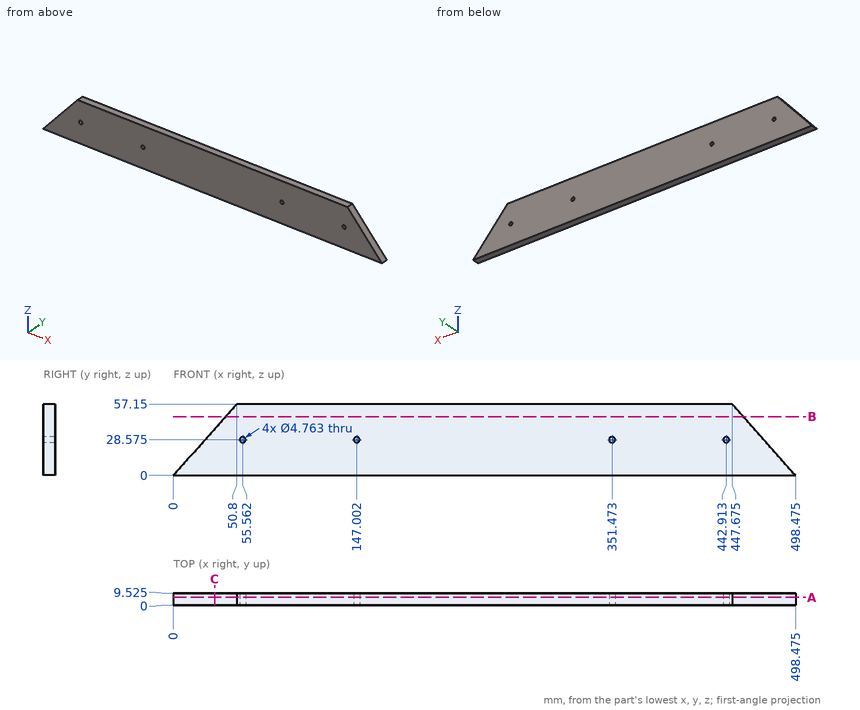
Input: dimensioned drawing with shaded views. Units: mm. Origin: part minimum x, y, z. Give positions to 0.01 mm unless a question says otherwise; leave off trailing zeros. Write each loop counter-clockwise with the first axis right and the second up, starting at its lowest first coordinate (ties: lowest second). Pieces come first, ordered by that corner, then holes. Notation, with made-up numbers: M -40,65 L -13,65 A14 ccw -13,86 Z; hole C -20.75,-21.75 d8. An arc over 180 degrees is marked long. Write item = value, one per line. Start each with the question number.
1) Cut plane A-A on y = 6.25. Count the separate pieces of the cut face and the enclosed holes in it, then the cut area to 3 significant figures.
2) Cut plane C-C on x = 33. Return the cut outline in (y, z) (1 decimal), then the cut area to 3 significant figures.
3) Material intervals for line 1 along X through (y, z) = (2.25, 37.5) (1 decimal); line 2 along X through (y, z) = (5, 22.5) (1 decimal); line 3 along Z through (x, y) = (43.5, 3) (1 decimal), sorted ascending. Write a range as [from, to].
4) First-contact query: pin 1 Ø1 at (y, z) = (1, 22) entering from -X; pin 2 Ø5.5 at (x, z) = (55.56, 28.58) entering from -Y; pin 3 Ø4 at (y, z) = (6.5, 19) entering from +X (1 decimal); pin 4 Ø5 at (y, z) = (5.5, 45) entering from -X. Flat tips, straight axial feed; report the tip coordinate or a pass-through.
5) Cut plane B-B on z = 47. Return the cut outline in (x, y) (1 decimal), then the cut area to 3 significant figures.
Solved:
q1.separate_pieces = 1
q1.enclosed_holes = 4
q1.area = 25,500 mm2
q2.outline = M 0,0 L 9.5,0 L 9.5,37.1 L 0,37.1 Z
q2.area = 354 mm2
q3.line_1 = [33.3, 465.1]
q3.line_2 = [20, 478.5]
q3.line_3 = [0, 48.9]
q4.pin_1 = 19.11
q4.pin_2 = 0
q4.pin_3 = 483.4
q4.pin_4 = 37.78
q5.outline = M 41.8,0 L 456.7,0 L 456.7,9.5 L 41.8,9.5 Z
q5.area = 3,950 mm2
